Input: part model. Units: mm. Frame: model coordinates. Give positions to 0.01 mm unless a question says otherwise; leave off trailing zeros. Order: outer loops, then holes, each group sorted by start corner. A loop starts at its lowest first (then second) coordinate and runs counter-clockwise, first axis right, second up. Notation, with made-up numbers: (71, 66) - (111, 66) arc R9 ccw to (111, 79) - close; hole circle Ø7 at (8, 78). An arc over 180 degrees is marked (long way). Use a Markdown table: item, result.
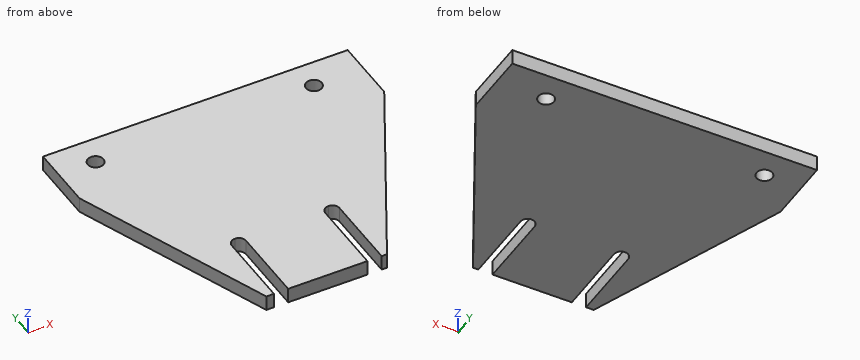
from build123d import *

# Parameters (mm, degrees)
F3_DEPTH = 3
F1_R     = 1.55
F4_DEPTH = 25
F5_DEPTH = 25


with BuildPart() as f3:
    # F0 (on Top) → F3 (new body)
    with BuildSketch(Plane.XY):
        Polygon((21.024429, 52), (-38.975571, 52), (-38.975571, 39), (-23.762762, 0), (0, 0), (21.024429, 39), align=None)
    extrude(amount=F3_DEPTH)

    # F1 (on Top) → F4 (cut)
    with BuildSketch(Plane.XY):
        with Locations((-31.737244, 46.35926)):
            Circle(F1_R)
        with Locations((11.262756, 46.35926)):
            Circle(F1_R)
    extrude(amount=F4_DEPTH, mode=Mode.SUBTRACT)

    # F2 (on face) → F5 (cut)
    with BuildSketch(Plane.XY):
        with BuildLine():
            Line((-3.852762, 15), (-3.852762, 0))
            Line((-3.852762, 0), (-2.452762, 0))
            Line((-2.452762, 0), (-1.052762, 0))
            Line((-1.052762, 0), (-1.052762, 15))
            ThreePointArc((-1.052762, 15), (-1.462812, 15.989949), (-2.452762, 16.4))
            ThreePointArc((-2.452762, 16.4), (-3.442711, 15.989949), (-3.852762, 15))
        make_face()
        with BuildLine():
            Line((-22.262762, 15), (-22.262762, 0))
            Line((-22.262762, 0), (-20.862762, 0))
            Line((-20.862762, 0), (-19.462762, 0))
            Line((-19.462762, 0), (-19.462762, 15))
            ThreePointArc((-19.462762, 15), (-19.872812, 15.989949), (-20.862762, 16.4))
            ThreePointArc((-20.862762, 16.4), (-21.852711, 15.989949), (-22.262762, 15))
        make_face()
    extrude(amount=F5_DEPTH, mode=Mode.SUBTRACT)


solid = f3.part
1. Pin query (flat end, axial travel): pin 1 (0.9 mm diameter, centred on y = 4.5, z = 2, fed in from +X); pin 2 (0.9 mm diameter, centred on y = 4, z = 2, fed in from -X); pin 3 (1.5 mm diameter, centred on y = 10, z = 2, fed in from -X). Return the tip coordinate at first contact, or that it passes through.
Response:
| item | result |
|---|---|
| pin 1 | stops at x = 2.67 |
| pin 2 | stops at x = -25.5 |
| pin 3 | stops at x = -27.96 |
2. Section query D-D (y = 27.5). Return loops of the section in (x, z).
Response:
| item | result |
|---|---|
| outline | (-34.49, 0) - (14.82, 0) - (14.82, 3) - (-34.49, 3) - close |
3. Section query A-A (y = 11.5). Return loops of the section in (x, z), then the cut area to 3 significant figures.
Response:
| item | result |
|---|---|
| outline | (-28.25, 0) - (-22.26, 0) - (-22.26, 3) - (-28.25, 3) - close; (-19.46, 0) - (-3.85, 0) - (-3.85, 3) - (-19.46, 3) - close; (-1.05, 0) - (6.2, 0) - (6.2, 3) - (-1.05, 3) - close |
| area | 86.5 mm^2 |
4. Material intervals for line 1 along X through (y, z) = (16, 1.35); line 2 along X through (y, z) = (7, 2.4); line 3 along Y through (x, z) = (6, 2.1), sorted ascending.
Response:
| item | result |
|---|---|
| line 1 | x = -30 to -21.84, -19.88 to -3.43, -1.47 to 8.63 |
| line 2 | x = -26.49 to -22.26, -19.46 to -3.85, -1.05 to 3.77 |
| line 3 | y = 11.13 to 52 |
5. Section query C-C (x = 2). Return loops of the section in (y, z).
Response:
| item | result |
|---|---|
| outline | (3.71, 0) - (52, 0) - (52, 3) - (3.71, 3) - close |
6. Section query B-B (z = 1.45). Return loops of the section in (x, y), then the cut area to 3 significant figures.
Response:
| item | result |
|---|---|
| outline | (-38.98, 39) - (-23.76, 0) - (-22.26, 0) - (-22.26, 15) arc R1.4 cw to (-20.86, 16.4) arc R1.4 cw to (-19.46, 15) - (-19.46, 0) - (-3.85, 0) - (-3.85, 15) arc R1.4 cw to (-2.45, 16.4) arc R1.4 cw to (-1.05, 15) - (-1.05, 0) - (0, 0) - (21.02, 39) - (21.02, 52) - (-38.98, 52) - close; hole circle Ø3.1 at (-31.74, 46.36); hole circle Ø3.1 at (11.26, 46.36) |
| area | 2,310 mm^2 |
